Part print with two shaded views. Sizes in mm from the minimum x, y, z corner. A direction names the side the tool comes from. Round coordinates to 2 decimals unless told otherwise and drop trailing zeros. Write each loop counter-clockwise with the first axis right and the second up, starting at its lowest first coordinate (ties: lowest second). Pieces come first, ordered by that corner, then holes. Notation, with made-up numbers: M -35.5,-17.5 L -28.5,-17.5 A6 ccw -28.5,-10.5 Z; hole C 0.25,65 d10. An arc over 180 degrees is marked long. Use one line per item in the form item = value. Start each with the question number.
Item 1: Which spindle directions (+Z, -Z, +X, -X, +Y, -Y) get a long thin tool onto all of the face, cutting with end or side? Do the marked faces 1, 2 and 3. Say none if no direction does.
Item 2: Cut at B-B, the plane x = 8.25. Give the cut face in (y, z), then the cut area to 3 significant figures.
Item 3: Probe L1, parallel to Z at x = 4.25, y = 6.75 (3 decimals); L2, parallel to X at y = 4.25, z = 44; L3, parallel to Z at x = 6.5, y = 7.25. List the from-to ranges inside material, lowest first.
Item 4: Cut at A-A, the plane z = 9. Give the cut face in (x, y) (3 decimals).
Item 5: Flat gauge pins, fed straight in: pin 1 Ø1 at (y, z) = (7, 65) entering from +X; pin 2 Ø2.5 at (x, y) = (3, 6.5) entering from -Z; pin 3 Ø3 at (x, z) = (4.445, 38.1) entering from -Y; pin 4 Ø3 at (y, z) = (2.5, 38.5) entering from -X. Where does each tip first touch, or does it go through?
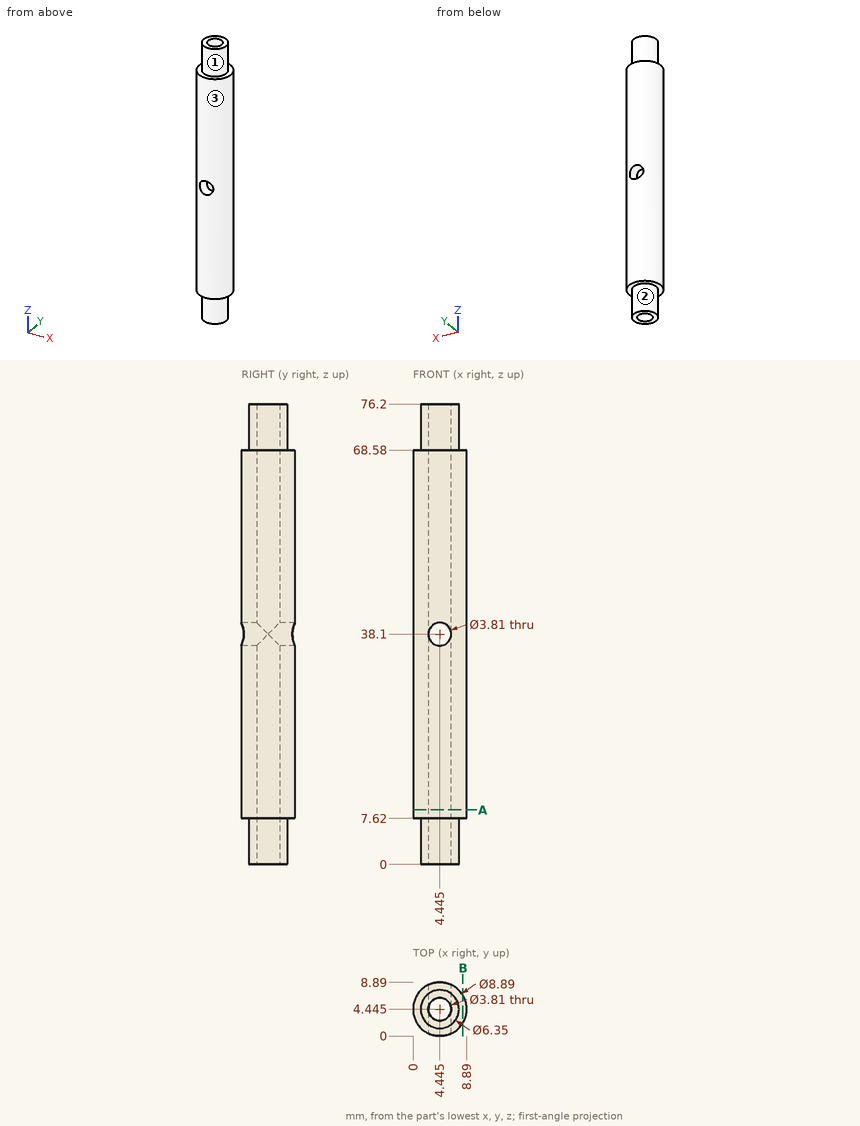
Model answer:
q1.face_1 = +Z
q1.face_2 = -Z
q1.face_3 = +Z, -Z
q2.outline = M 2.15,7.62 L 6.74,7.62 L 6.74,68.58 L 2.15,68.58 Z
q2.area = 280 mm²
q3.L1 = 0 to 36.205, 39.995 to 76.2
q3.L2 = 0 to 2.55, 6.34 to 8.89
q3.L3 = 7.62 to 68.58
q4.outline = C 4.445,4.445 d8.89; hole C 4.445,4.445 d3.81
q5.pin_1 = 8.39
q5.pin_2 = 0
q5.pin_3 = through
q5.pin_4 = 0.02
